Answer from the drawing. Dimensions are ordinates in mm from the lowest x, y and z of the part. A direction names the side the tool comes from. Give positions to 0.01 mm unless a question says otherwise; leave off trailing zeros. Order: outer loops, then holes, each group sorted by start corner. A loop starts at its lowest first (then second) coordinate and runs counter-clockwise, first axis right, second up.
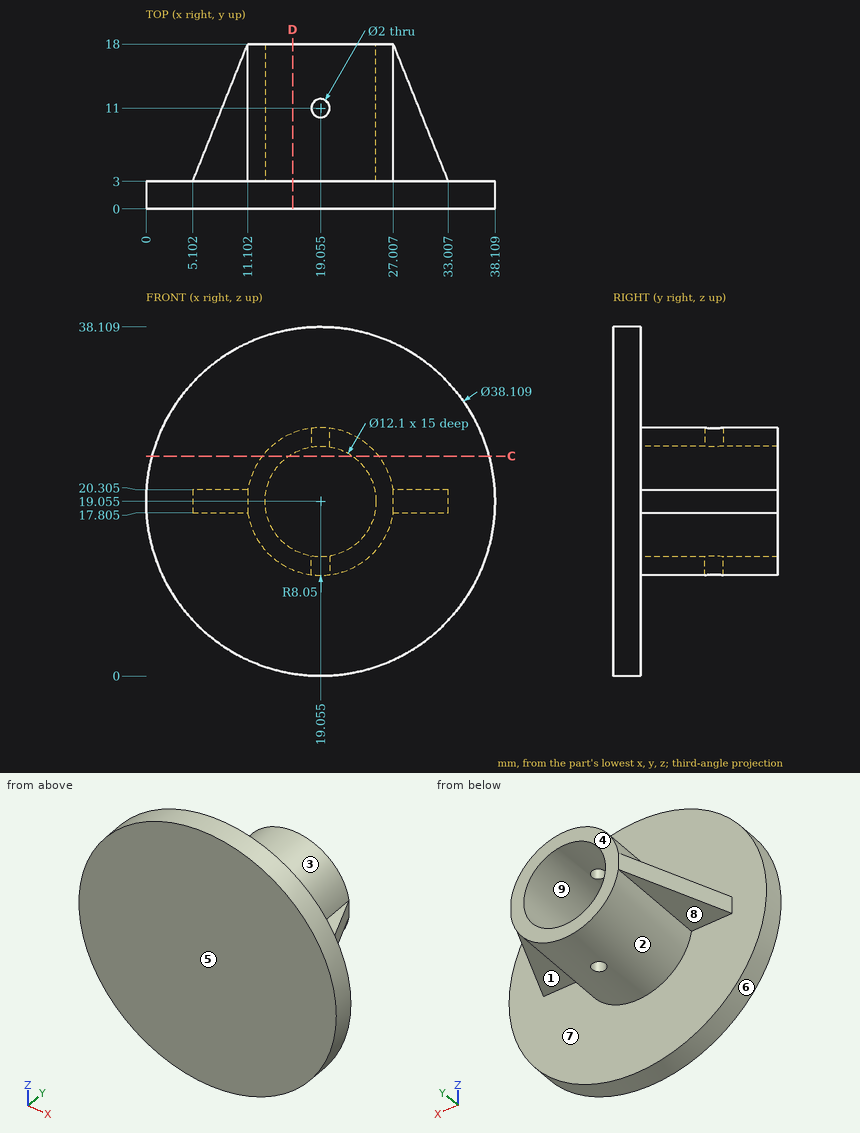
1) The part is cut by section C-C on z = 24. Determine the outline of the cut face in (x, y).
Final values:
outline: (0.65, 0) - (37.46, 0) - (37.46, 3) - (25.41, 3) - (25.41, 18) - (22.54, 18) - (22.54, 3) - (15.57, 3) - (15.57, 18) - (12.7, 18) - (12.7, 3) - (0.65, 3) - close
2) A tool of negligible diameter and unlimited length cuts with its end or side. For the marked faces 1, 2, 3, 4 and 5, from which of +Z, -Z, +X, -X, +Y, -Y can it reach the whole face along a straight path? Write none if from no direction.
Final values:
face 1: -Z, +X, +Y
face 2: -Z, +Y
face 3: +Z, +Y
face 4: +Z, -Z, +X, -X, +Y
face 5: +Z, -Z, +X, -X, -Y
3) The part is cut by section D-D on x = 16. Determine the outline of the cut face in (y, z).
Final values:
outline: (0, 0.25) - (3, 0.25) - (3, 11.61) - (18, 11.61) - (18, 13.83) - (3, 13.83) - (3, 24.28) - (18, 24.28) - (18, 26.5) - (3, 26.5) - (3, 37.86) - (0, 37.86) - close
4) Given pin 1 (1.2 mm diameter, centred on x = 19.05, y = 11, fed in from -Z); pin 2 (1.8 mm diameter, centred on x = 8.5, y = 11.5, fed in from -Z) (1 decimal); pin 3 (8 mm diameter, centred on y = 13.5, z = 15.5, fed in from -X) (1 decimal); pin 4 (2 mm diameter, centred on y = 9.5, z = 20, fed in from +X), each flat-ended and moving along its own axis, determine where each tip first touches the part or whether it passes through.
Final values:
pin 1: passes through
pin 2: stops at z = 17.8
pin 3: stops at x = 8
pin 4: stops at x = 30.81
5) For a pull along Z with two mould halves and no side action, classify the marked faces 6, 7, 8 and 9 as released by +Z, released by -Z, zero draft, split by the parting line, or undercut.
Final values:
face 6: split by the parting line
face 7: zero draft
face 8: released by -Z
face 9: undercut
6) Consider L1, parallel to Y at x = 24.5, z = 9.5; L2, parallel to Z at x = 8.5, y = 5.25 (1 decimal); L3, parallel to X at y = 11, z = 12.15 (1 decimal). Determine where each line is inside the solid, lowest interval first.
Final values:
L1: y = 0 to 3
L2: z = 17.8 to 20.3
L3: x = 14.9 to 18.1, 20.1 to 23.2
